For this review, use the dimensioned drawing (mm, ordinates from the lowest corner) and the shaded views. A direction names the side the tool comes from. Coordinates: 2 decimals unless noted, no trailing zeros. Order: outer loops, then holes, each group sorted by start corner. A loop starts at its lowest first (then second) coordinate and runs counter-clockwise, first axis right, second up. Notation, with made-up numbers: M 18.5,-36.5 L 23.5,-36.5 A26 ccw 23.5,-7.5 Z; hole C -4,32.5 d4. An arc over 180 degrees is marked long. Use one line per item in the form item = value. Start each with the question number.
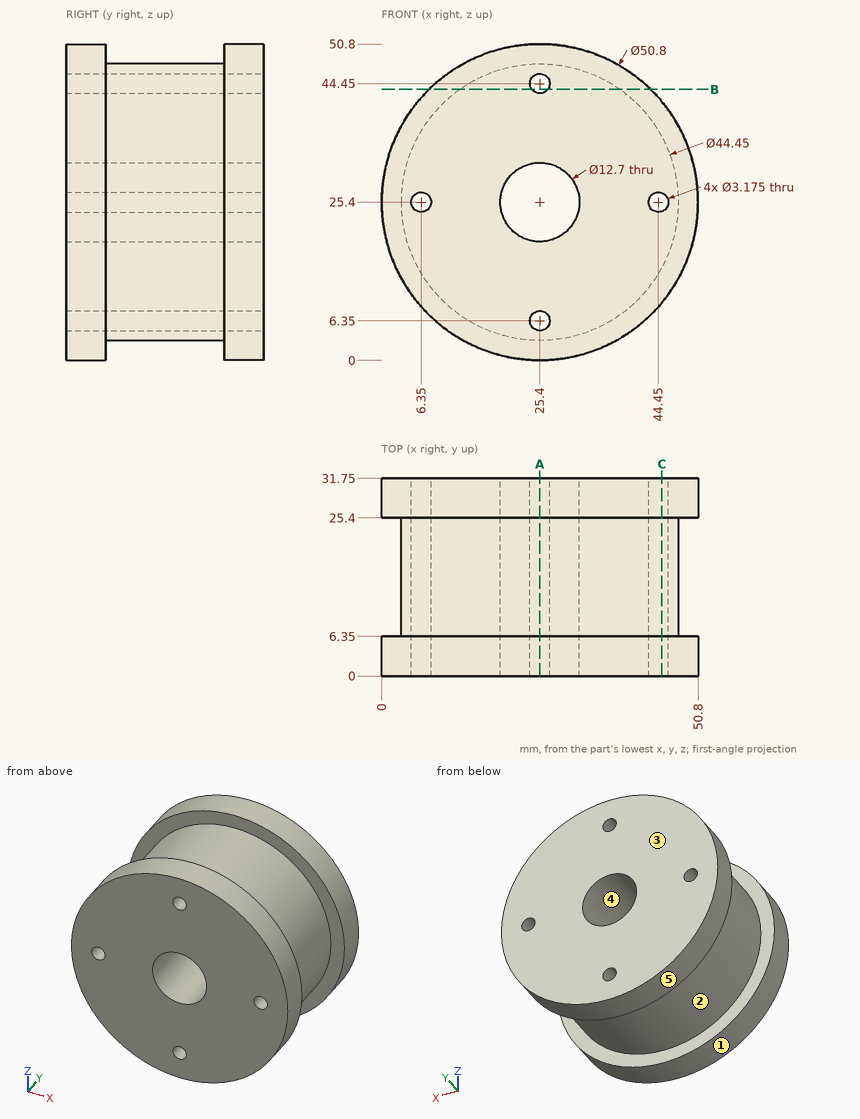
1. For pin 1 Ø1.5 at (x, y) = (14.5, 20) entering from +Z; pin 2 Ø1.9 at (x, z) = (6.35, 25.4) entering from +Y; pin 3 Ø5 at (x, y) = (42, 7) entering from +Z; pin 4 Ø8 at (x, y) = (13.5, 26) entering from +Z, all flat-tipped, find the tip position at first contact; note any pin that passes through.
2. Consider section A-A, the plane x = 25.4. Give the number of separate pieces and of enclosed holes in the cut face, plus the area to 3 significant figures.
3. To check wall thickness, follow line 1 (Y direction, x = 44, z = 38); line 2 (Z direction, x = 25, y = 10); line 3 (Z direction, x = 26, y = 11). State the ranges of each line that lie inside material, in increasing order.
4. Tool access review of the marked faces 1 and 2: name each direction out of +Z, -Z, +X, -X, +Y, -Y from which nothing blocks a thin tool from reaching the whole face with its end or side.
5. The part is to be moulded in two halves that separate along Z. For the marked faces 3, 4 and 5, say which applies: pulls with the +Z half, pulls with the -Z half, needs draft (parallel to the pull), parting line crosses it, or undercut.
6. Consider section B-B, the plane z = 43.5. Write out the cut boundary in (x, y), plus the area to 3 significant figures.
7. Consider section C-C, the plane x = 45. Write out the cut boundary in (y, z).
Answers follow:
q1.pin_1 = 45.17
q1.pin_2 = through
q1.pin_3 = 46.47
q1.pin_4 = 49.54
q2.separate_pieces = 4
q2.enclosed_holes = 0
q2.area = 887 mm²
q3.line_1 = 0 to 6.35, 25.4 to 31.75
q3.line_2 = 3.18 to 4.81, 7.89 to 19.06, 31.74 to 42.91, 45.99 to 47.62
q3.line_3 = 3.18 to 4.88, 7.82 to 19.08, 31.72 to 42.98, 45.92 to 47.62
q4.face_1 = +Y, -Y
q4.face_2 = none
q5.face_3 = needs draft
q5.face_4 = undercut
q5.face_5 = parting line crosses it
q6.outline = M 7.58,0 L 24.13,0 L 24.13,31.75 L 7.58,31.75 L 7.58,25.4 L 12.5,25.4 L 12.5,6.35 L 7.58,6.35 Z; M 26.67,0 L 43.22,0 L 43.22,6.35 L 38.3,6.35 L 38.3,25.4 L 43.22,25.4 L 43.22,31.75 L 26.67,31.75 Z
q6.area = 863 mm²
q7.outline = M 0,9.24 L 6.35,9.24 L 6.35,14.92 L 25.4,14.92 L 25.4,9.24 L 31.75,9.24 L 31.75,23.91 L 0,23.91 Z; M 0,26.89 L 31.75,26.89 L 31.75,41.56 L 25.4,41.56 L 25.4,35.88 L 6.35,35.88 L 6.35,41.56 L 0,41.56 Z
